Could you check a few things on this model? Use its own coordinates, in mm. Coordinates: 2 decimals unless noted, no trailing zeros. Loops run counter-clockwise (first coordinate to the right, second up) from the corner with the lowest first, then second, coordinate; pieces in that order, holes last. Notation, with made-up numbers: (65, 38.5) - (106, 38.5) arc R13 cw to (106, 45.5) - close; hole circle Ø1 at (-29.5, 45). An arc over 180 degrees is marked (long way). Use CSV: the item, a comma, the result in double quotes.
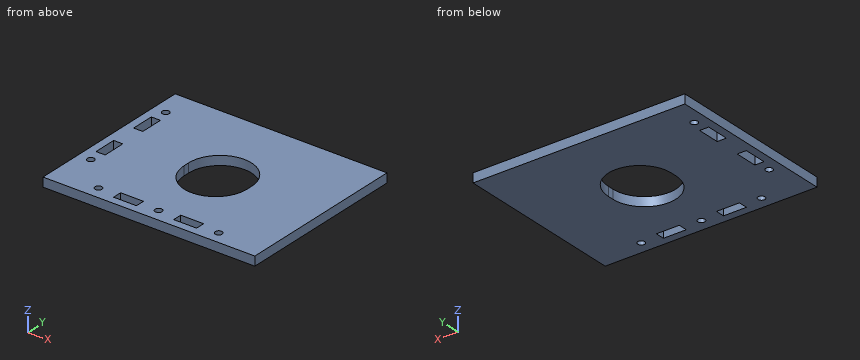
from build123d import *

# Parameters (mm, degrees)
MODEL_W             = 185
MODEL_H             = 150
MODEL_R             = 3.05
MODEL_W_2           = 20
MODEL_H_2           = 8
MODEL_W_3           = 8
MODEL_H_3           = 20
BOSS_EXTRUDE1_DEPTH = 8


with BuildPart() as part:
    # Model → Boss-Extrude1 (new body)
    with BuildSketch(Plane.XY):
        with Locations((77.5, 60)):
            Rectangle(MODEL_W, MODEL_H)
        with Locations((130, -4)):
            Circle(MODEL_R, mode=Mode.SUBTRACT)
        with Locations((25, -4)):
            Circle(MODEL_R, mode=Mode.SUBTRACT)
        with Locations((-4, 25)):
            Circle(MODEL_R, mode=Mode.SUBTRACT)
        with Locations((-4, 110)):
            Circle(MODEL_R, mode=Mode.SUBTRACT)
        with Locations((77.5, -4)):
            Circle(MODEL_R, mode=Mode.SUBTRACT)
        with Locations((103.75, -4)):
            Rectangle(MODEL_W_2, MODEL_H_2, mode=Mode.SUBTRACT)
        with BuildLine():
            Line((52.5, 57.5), (52.5, 62.5))
            ThreePointArc((52.5, 62.5), (80, 90), (107.5, 62.5))
            Line((107.5, 62.5), (107.5, 57.5))
            ThreePointArc((107.5, 57.5), (80, 30), (52.5, 57.5))
        make_face(mode=Mode.SUBTRACT)
        with Locations((51.25, -4)):
            Rectangle(MODEL_W_2, MODEL_H_2, mode=Mode.SUBTRACT)
        with Locations((-4, 88.75)):
            Rectangle(MODEL_W_3, MODEL_H_3, mode=Mode.SUBTRACT)
        with Locations((-4.13466, 46.25)):
            Rectangle(MODEL_W_3, MODEL_H_3, mode=Mode.SUBTRACT)
    extrude(amount=BOSS_EXTRUDE1_DEPTH)


solid = part.part
(1) Suppose I cut it at D-D (y = 110). Write out the boundary of the cut face in (x, z).
Computed:
outline,"(-15, 0) - (-7.05, 0) - (-7.05, 8) - (-15, 8) - close; (-0.95, 0) - (170, 0) - (170, 8) - (-0.95, 8) - close"
(2) Please list where these lines run through material, in increasing order: line 1 (Y direction, x = -4, z = 5); line 2 (Y direction, x = 25, z = 3.25); line 3 (X direction, y = 95, z = 2).
Computed:
line 1,"y = -15 to 21.95, 28.05 to 36.25, 56.25 to 78.75, 98.75 to 106.95, 113.05 to 135"
line 2,"y = -15 to -7.05, -0.95 to 135"
line 3,"x = -15 to -8, 0 to 170"
(3) Suppose I cut it at A-A (x = 25). Write out the boundary of the cut face in (y, z), plus the area to 3 significant figures.
Computed:
outline,"(-15, 0) - (-7.05, 0) - (-7.05, 8) - (-15, 8) - close; (-0.95, 0) - (135, 0) - (135, 8) - (-0.95, 8) - close"
area,"1,150 mm²"
(4) Will this pin go through, and if not, where does the flat tip stop? pin 1 (5.5 mm diameter, centred on x = 130, y = -4, fed in from -Z).
Computed:
pin 1,"passes through"
(5) Suppose I cut it at C-C (x = -4). Write out the boundary of the cut face in (y, z).
Computed:
outline,"(-15, 0) - (21.95, 0) - (21.95, 8) - (-15, 8) - close; (28.05, 0) - (36.25, 0) - (36.25, 8) - (28.05, 8) - close; (56.25, 0) - (78.75, 0) - (78.75, 8) - (56.25, 8) - close; (98.75, 0) - (106.95, 0) - (106.95, 8) - (98.75, 8) - close; (113.05, 0) - (135, 0) - (135, 8) - (113.05, 8) - close"
(6) Suppose I cut it at B-B (y = -4). Write out the boundary of the cut face in (x, z), plus the area to 3 significant figures.
Computed:
outline,"(-15, 0) - (21.95, 0) - (21.95, 8) - (-15, 8) - close; (28.05, 0) - (41.25, 0) - (41.25, 8) - (28.05, 8) - close; (61.25, 0) - (74.45, 0) - (74.45, 8) - (61.25, 8) - close; (80.55, 0) - (93.75, 0) - (93.75, 8) - (80.55, 8) - close; (113.75, 0) - (126.95, 0) - (126.95, 8) - (113.75, 8) - close; (133.05, 0) - (170, 0) - (170, 8) - (133.05, 8) - close"
area,"1,010 mm²"
